from build123d import *

# Parameters (mm, degrees)
CUT_EXTRUDE_3_DEPTH = 11
SKETCH_3_R          = 1.25
CUT_EXTRUDE_4_DEPTH = 13


with BuildPart() as part:
    # 草图1 → 旋转1 (revolve)
    with BuildSketch(Plane.XY, mode=Mode.PRIVATE) as revolve_1_sk:
        Polygon((-29.173795435, 0), (-29.173795435, 7.650126796), (-25.287235841, 7.650126796), (-25.287235841, 11.290701606), (-22.473795435, 11.290701606), (-22.473795435, 12.1), (-3.423795435, 12.1), (-3.423795435, 12.4), (15.326204565, 12.4), (15.326204565, 3.5), (18.026204565, 3.5), (18.026204565, 1.5), (29.026204565, 1.5), (29.026204565, 0), align=None)
    revolve(revolve_1_sk.sketch.rotate(Axis((-38.029247675, 0, 0), (1, 0, 0)), 90), axis=Axis((-38.029247675, 0, 0), (1, 0, 0)))

    # 草图2 → 切除-拉伸3 (cut)
    with BuildSketch(Plane(origin=(29.026204565, 0, 0), x_dir=(0, 0, -1), z_dir=(1, 0, 0))):
        Polygon((-49.186248705, 1), (-1.118033989, 1), (1.118033989, 1), (49.186248705, 1), (49.186248705, 97.136429433), (-49.186248705, 97.136429433), align=None)
    extrude(amount=-CUT_EXTRUDE_3_DEPTH, mode=Mode.SUBTRACT)

    # 草图3 → 切除-拉伸4 (cut)
    with BuildSketch(Plane(origin=(15.326204565, 0, 0), x_dir=(0, 0, -1), z_dir=(1, 0, 0))):
        with Locations((-8.5, 0)):
            Circle(SKETCH_3_R)
        with Locations(Location((8.5, 0, 0), (0, 0, 180))):
            Circle(SKETCH_3_R)
    extrude(amount=-CUT_EXTRUDE_4_DEPTH, mode=Mode.SUBTRACT)


solid = part.part
Source: CAD feature listing. Evaluate the final solid. Frame: model axes, mm. A direction names the side the tool comes from. Round coordinates to 2 decimals unless told otherwise and drop trailing zeros. Loops run counter-clockwise (first coordinate to the right, second up) from the corner with the lowest first, then second, coordinate; pieces in that order, holes last. Notation, with made-up numbers: (-7.5, 56.25) -> (5.5, 56.25) arc R27 ccw to (5.5, 76.25) -> close; hole circle Ø6 at (66.25, 73.5). An arc over 180 degrees is marked (long way). Answer as a JSON object with one key per item and string values. Group by question number.
Q1. Contact query for flat-ended pins moving along their axis: P1, Ø1.5, axis at y = 0, z = -8.5, coming from the -X side; P2, Ø7.5, axis at y = -5, z = -6, coming from the +X side; P3, Ø2, axis at y = 2, z = 1.5, coming from the +X side. Output: stop coordinate, or through.
Q2. Section query B-B (z = 0). Output: boundary loops of the cut face in (x, y).
Q3. Section query D-D (z = -5.75). Output: boundary loops of the cut face in (x, y), plus the area to 3 significant figures.
Q4. Access query for faces 5 (the cylindrical face through (-12.815, -3.635, 11.541)), 6 (the flat face through (24, 1, 0)), 7 (the cylindrical face through (23.6, -1.5, 0)). Directions: +Z, -Z, +X, -X, +Y, -Y. A direction counts if a zero-diameter tool reaches every point of the face in a straight line with its end or side. Return the directions, or none.
Q5. Ray query, line 1 (X direction, y = -1.75, z = -0.25); line 2 (X direction, y = -3.5, z = 6.5); line 3 (Y direction, x = 5, z = 8.5). Return the intervals inside material, ascending. Write a range as from..to.
Q6. Mould query, pull axis Z, two halves, no side actions, for faces 1 (the cylindrical face through (6.08, -3.72, 11.83)), 2 (the cylindrical face through (8.92, 0.05, 9.75)), 3 (the cylindrical face through (8.92, -0.05, -9.75)), 4 (the flat face through (-25.287, 7.4, 2.7)). Classes: pulls with the +Z half, pulls with the -Z half, needs draft (parallel to the pull), parting line crosses it, or undercut.
Q7. Section query C-C (x = 6.5). Output: boundary loops of the cut face in (y, z), plus the area to 3 significant figures.
Completed:
{
 "1": {"P1": "x = -25.29", "P2": "x = 15.33", "P3": "x = 18.03"},
 "2": {"outline": "(-29.17, -7.65) -> (-25.29, -7.65) -> (-25.29, -11.29) -> (-22.47, -11.29) -> (-22.47, -12.1) -> (-3.42, -12.1) -> (-3.42, -12.4) -> (15.33, -12.4) -> (15.33, -3.5) -> (18.03, -3.5) -> (18.03, -1.5) -> (29.03, -1.5) -> (29.03, 1) -> (18.03, 1) -> (18.03, 3.5) -> (15.33, 3.5) -> (15.33, 12.4) -> (-3.42, 12.4) -> (-3.42, 12.1) -> (-22.47, 12.1) -> (-22.47, 11.29) -> (-25.29, 11.29) -> (-25.29, 7.65) -> (-29.17, 7.65) -> close"},
 "3": {"outline": "(-29.17, -5.05) -> (-25.29, -5.05) -> (-25.29, -9.72) -> (-22.47, -9.72) -> (-22.47, -10.65) -> (-3.42, -10.65) -> (-3.42, -10.99) -> (15.33, -10.99) -> (15.33, 10.99) -> (-3.42, 10.99) -> (-3.42, 10.65) -> (-22.47, 10.65) -> (-22.47, 9.72) -> (-25.29, 9.72) -> (-25.29, 5.05) -> (-29.17, 5.05) -> close", "area": "912 mm²"},
 "4": {"face 5": "-X", "face 6": "+Z, -Z, +X, +Y", "face 7": "+X"},
 "5": {"line 1": "-29.17..18.03", "line 2": "-29.17..15.33", "line 3": "-9.03..-1.25, 1.25..9.03"},
 "6": {"face 1": "parting line crosses it", "face 2": "undercut", "face 3": "undercut", "face 4": "needs draft"},
 "7": {"outline": "circle Ø24.8 at (0, 0); hole circle Ø2.5 at (0, -8.5); hole circle Ø2.5 at (0, 8.5)", "area": "473 mm²"}
}
